from build123d import *

# Parameters (mm, degrees)
ESQUISSE1_W                         = 48.006
ESQUISSE1_H                         = 42.242296956
BOSS_EXTRU_1_DEPTH                  = 42.242296957
ESQUISSE2_R                         = 11
BOSS_EXTRU_2_DEPTH                  = 2.286
ESQUISSE3_R                         = 2.5
BOSS_EXTRU_3_DEPTH                  = 22.352
ENL_V_START                         = -14.478
ENL_V_MAT_EXTRU_1_DEPTH             = 14.478
ESQUISSE5_W                         = 7.62
ESQUISSE5_H                         = 6.35
ENL_V_MAT_EXTRU_2_DEPTH             = 2.54
ESQUISSE6_W                         = 0.635
ESQUISSE6_H                         = 25.4
ESQUISSE7_W                         = 0.635
ESQUISSE7_H                         = 25.4
ESQUISSE8_W                         = 0.635
ESQUISSE8_H                         = 25.4
ESQUISSE9_W                         = 0.635
ESQUISSE9_H                         = 25.4
D_GAGEMENT_M81_D                    = 9.017
D_GAGEMENT_M81_DEPTH                = 4.191
DIAM_TRE_DU_PER_AGE_4_0_4_1_D       = 4
DIAM_TRE_DU_PER_AGE_4_0_4_1_DEPTH   = 4.191
DIAM_TRE_DU_PER_AGE_3_5_3_5_1_D     = 3.5
DIAM_TRE_DU_PER_AGE_3_5_3_5_1_DEPTH = 4.572
CHANFREIN1_SIZE                     = 0.254
CHANFREIN2_SIZE                     = 2.54
CHANFREIN3_SIZE                     = 0.508
CONG_1_R                            = 0.381


with BuildPart() as part:
    # Esquisse1 → Boss.-Extru.1 (new body)
    with BuildSketch(Plane(origin=(21.121148478, 0, 0), x_dir=(0, 0, -1), z_dir=(1, 0, 0))):
        with Locations((24.003, 0)):
            Rectangle(ESQUISSE1_W, ESQUISSE1_H)
    extrude(amount=-BOSS_EXTRU_1_DEPTH)

    # Esquisse2 → Boss.-Extru.2 (add)
    with BuildSketch(Plane.XY):
        Circle(ESQUISSE2_R)
    extrude(amount=BOSS_EXTRU_2_DEPTH)

    # Esquisse3 → Boss.-Extru.3 (add)
    with BuildSketch(Plane.XY.offset(2.286)):
        Circle(ESQUISSE3_R)
    extrude(amount=BOSS_EXTRU_3_DEPTH)

    # Esquisse4 → Enlèv. mat.-Extru.1 (cut)
    with BuildSketch(Plane.XY.offset(24.638).offset(ENL_V_START)):
        with BuildLine():
            Line((-1.5, 2), (1.5, 2))
            ThreePointArc((1.5, 2), (0, 2.5), (-1.5, 2))
        make_face()
    extrude(amount=ENL_V_MAT_EXTRU_1_DEPTH, mode=Mode.SUBTRACT)

    # Esquisse5 → Enlèv. mat.-Extru.2 (cut)
    with BuildSketch(Plane(origin=(0, 21.121148478, 0), x_dir=(-1, 0, 0), z_dir=(0, 1, 0))):
        with Locations((0, -41.91)):
            Rectangle(ESQUISSE5_W, ESQUISSE5_H)
    extrude(amount=-ENL_V_MAT_EXTRU_2_DEPTH, mode=Mode.SUBTRACT)

    # Esquisse6 → Révolution1 (revolve)
    with BuildSketch(Plane(origin=(0, 0, -43.815), x_dir=(-1, 0, 0), z_dir=(0, 0, -1)), mode=Mode.PRIVATE) as r_volution1_sk:
        with Locations((-2.0955, 31.281148478)):
            Rectangle(ESQUISSE6_W, ESQUISSE6_H)
    revolve(r_volution1_sk.sketch.rotate(Axis((1.778, 18.581148478, -43.815), (0, 1, 0)), 270), axis=Axis((1.778, 18.581148478, -43.815), (0, 1, 0)))

    # Esquisse7 → Révolution2 (revolve)
    with BuildSketch(Plane(origin=(0, 0, -40.513), x_dir=(-1, 0, 0), z_dir=(0, 0, -1)), mode=Mode.PRIVATE) as r_volution2_sk:
        with Locations((-2.0955, 31.281148478)):
            Rectangle(ESQUISSE7_W, ESQUISSE7_H)
    revolve(r_volution2_sk.sketch.rotate(Axis((1.778, 18.581148478, -40.513), (0, 1, 0)), 270), axis=Axis((1.778, 18.581148478, -40.513), (0, 1, 0)))

    # Esquisse8 → Révolution3 (revolve)
    with BuildSketch(Plane(origin=(0, 0, -43.815), x_dir=(-1, 0, 0), z_dir=(0, 0, -1)), mode=Mode.PRIVATE) as r_volution3_sk:
        with Locations((1.4605, 31.281148478)):
            Rectangle(ESQUISSE8_W, ESQUISSE8_H)
    revolve(r_volution3_sk.sketch.rotate(Axis((-1.778, 18.581148478, -43.815), (0, 1, 0)), 270), axis=Axis((-1.778, 18.581148478, -43.815), (0, 1, 0)))

    # Esquisse9 → Révolution4 (revolve)
    with BuildSketch(Plane(origin=(0, 0, -40.513), x_dir=(-1, 0, 0), z_dir=(0, 0, -1)), mode=Mode.PRIVATE) as r_volution4_sk:
        with Locations((1.4605, 31.281148478)):
            Rectangle(ESQUISSE9_W, ESQUISSE9_H)
    revolve(r_volution4_sk.sketch.rotate(Axis((-1.778, 18.581148478, -40.513), (0, 1, 0)), 270), axis=Axis((-1.778, 18.581148478, -40.513), (0, 1, 0)))

    # Dégagement M81
    with Locations(Plane(origin=(0, 0, -48.006), x_dir=(-1, 0, 0), z_dir=(0, 0, -1))):
        with Locations((0, 0)):
            Hole(D_GAGEMENT_M81_D / 2, depth=D_GAGEMENT_M81_DEPTH)

    # Diamètre du perçage Ø4.0 (4)1
    with Locations(Plane(origin=(0, 0, -48.006), x_dir=(-1, 0, 0), z_dir=(0, 0, -1))):
        with Locations((15.5, 15.5), (-15.5, -15.5), (15.5, -15.5), (-15.5, 15.5)):
            Hole(DIAM_TRE_DU_PER_AGE_4_0_4_1_D / 2, depth=DIAM_TRE_DU_PER_AGE_4_0_4_1_DEPTH)

    # Diamètre du perçage Ø3.5 (3.5)1
    with Locations(Plane.XY):
        with Locations((-15.5, 15.5), (15.5, 15.5), (-15.5, -15.5), (15.5, -15.5)):
            Hole(DIAM_TRE_DU_PER_AGE_3_5_3_5_1_D / 2, depth=DIAM_TRE_DU_PER_AGE_3_5_3_5_1_DEPTH)

    # Chanfrein1
    chanfrein1_edges = [part.edges().sort_by_distance(p)[0] for p in [
        (-11, 0, 2.286),
        (-1.118033989, -2.236067977, 24.638),
        (0, 2, 24.638),
        (-4.5085, 0, -48.006),
        (13.5, 15.5, -48.006),
        (-17.5, -15.5, -48.006),
        (13.5, -15.5, -48.006),
        (-17.5, 15.5, -48.006),
        (17.25, -15.5, 0),
        (-13.75, -15.5, 0),
        (17.25, 15.5, 0),
        (-13.75, 15.5, 0),
    ]]
    chamfer(chanfrein1_edges, length=CHANFREIN1_SIZE)

    # Chanfrein2
    chanfrein2_edges = [part.edges().sort_by_distance(p)[0] for p in [
        (-21.121148478, -21.121148478, -24.003),
        (-21.121148478, 21.121148478, -24.003),
        (21.121148478, -21.121148478, -24.003),
        (21.121148478, 21.121148478, -24.003),
    ]]
    chamfer(chanfrein2_edges, length=CHANFREIN2_SIZE)

    # Chanfrein3
    chanfrein3_edges = [part.edges().sort_by_distance(p)[0] for p in [
        (0, 21.121148478, 0),
        (21.121148478, 0, 0),
        (-21.121148478, 0, 0),
        (0, -21.121148478, 0),
        (19.851148478, -19.851148478, 0),
        (19.851148478, 19.851148478, 0),
        (-19.851148478, -19.851148478, 0),
        (-19.851148478, 19.851148478, 0),
    ]]
    chamfer(chanfrein3_edges, length=CHANFREIN3_SIZE)

    # Congé1
    cong_1_edges = [part.edges().sort_by_distance(p)[0] for p in [
        (0, 21.121148478, -48.006),
        (-21.121148478, 0, -48.006),
        (21.121148478, 0, -48.006),
        (0, -21.121148478, -48.006),
        (19.851148478, -19.851148478, -48.006),
        (19.851148478, 19.851148478, -48.006),
        (-19.851148478, -19.851148478, -48.006),
        (-19.851148478, 19.851148478, -48.006),
    ]]
    fillet(cong_1_edges, radius=CONG_1_R)


solid = part.part
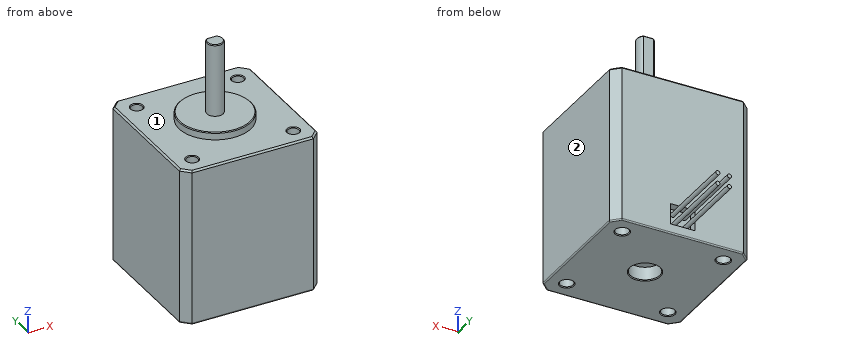
Design review of the part built by this model. Coordinates are the model's own, in mm. Face numbers are marked on the shaded views. A direction names the side the tool comes from. Give positions to 0.01 mm unless a question says otherwise; leave off trailing zeros. Order: outer loops, then holes, each group sorted by start corner. A loop starts at its lowest first (then second) coordinate and runs counter-clockwise, first axis right, second up. Notation, with made-up numbers: (76.5, -38.5) - (100.5, -38.5) arc R16 cw to (100.5, -7.5) - close; hole circle Ø7 at (25, 49.5). An arc over 180 degrees is marked (long way). Write item = value, one per line. Start each with the question number.
Q1. Tool access review of the marked faces 1 and 2: name each direction out of +Z, -Z, +X, -X, +Y, -Y from which nothing blocks a thin tool from reaching the whole face with its end or side.
Q2. To check wall thickness, follow L1, parallel to Y at x = -15.5, z = -2; L2, parallel to Y at x = 15.5, z = -45.1; L3, parallel to Y at x = 0, z = -44. State the ranges of each line that lie inside material, in increasing order. Write a range as from..to.
Q3. Clearance check with flat-ended pins moving along their axes: pin 1 Ø1 at (x, z) = (-9.5, -22.5) entering from +Y; pin 2 Ø5 at (x, y) = (-15.5, 15.5) entering from +Z; pin 3 Ø10 at (x, y) = (-12, 7) entering from +Z; pin 4 Ø10 at (y, z) = (-8, 2.5) entering from -X. State where each tip first meets the part, or that it passes through.
Q4. We need section C-C on z = -30.5. State the section outline as (x, y) points, plus the area to 3 significant figures.
Q5. We need section D-D on y = 25.5. State the section outline as (x, z) points (3 decimals).
Working result:
q1.face_1 = +Z
q1.face_2 = +Z, -Z, +X, +Y, -Y
q2.L1 = -21.12..-17.25, -13.75..13.75, 17.25..21.12
q2.L2 = -21.12..-17.5, -13.5..13.5, 17.5..21.12
q2.L3 = -21.12..-4.51, 4.51..18.58
q3.pin_1 = 21.12
q3.pin_2 = 0
q3.pin_3 = 2.29
q3.pin_4 = -21.12
q4.outline = (-21.12, -18.58) - (-18.58, -21.12) - (18.58, -21.12) - (21.12, -18.58) - (21.12, 18.58) - (18.58, 21.12) - (-18.58, 21.12) - (-21.12, 18.58) - close
q4.area = 1,770 mm²
q5.outline = circle Ø1.27 at (-1.778, -43.815); circle Ø1.27 at (-1.778, -40.513); circle Ø1.27 at (1.778, -43.815); circle Ø1.27 at (1.778, -40.513)
